```python
from build123d import *

# Parameters (mm, degrees)
F0_W      = 100
F0_H      = 200
F1_DEPTH  = 20
F3_DEPTH  = 10
F5_DEPTH  = 10
F6_R      = 45
F6_R_2    = 30
F7_DEPTH  = 10
F8_R      = 30
F9_DEPTH  = 32
F11_D     = 10
F11_DEPTH = 15
F11_TIP   = 3.0043030951


with BuildPart() as f1:
    # F0 (on Front) → F1 (new body)
    with BuildSketch(Plane.XZ):
        Rectangle(F0_W, F0_H)
    extrude(amount=F1_DEPTH)

    # F2 (on face) → F3 (cut)
    with BuildSketch(Plane(origin=(0, 0, 0), x_dir=(-1, 0, 0), z_dir=(0, 1, 0))):
        with BuildLine():
            ThreePointArc((-28, -60), (-36.4852813742, -63.5147186258), (-40, -72))
            Line((-40, -72), (-40, -78))
            ThreePointArc((-40, -78), (-36.4852813742, -86.4852813742), (-28, -90))
            Line((-28, -90), (28, -90))
            ThreePointArc((28, -90), (36.4852813742, -86.4852813742), (40, -78))
            Line((40, -78), (40, -72))
            ThreePointArc((40, -72), (36.4852813742, -63.5147186258), (28, -60))
            Line((28, -60), (-28, -60))
        make_face()
    extrude(amount=-F3_DEPTH, mode=Mode.SUBTRACT)

    # F4 (on face) → F5 (join)
    with BuildSketch(Plane(origin=(0, 0, 0), x_dir=(-1, 0, 0), z_dir=(0, 1, 0))):
        with BuildLine():
            Line((-48, 45.029), (-48, -38))
            ThreePointArc((-48, -38), (-45.0710678119, -45.0710678119), (-38, -48))
            Line((-38, -48), (38, -48))
            ThreePointArc((38, -48), (45.0710678119, -45.0710678119), (48, -38))
            Line((48, -38), (48, 45.029))
            ThreePointArc((48, 45.029), (47.0866406093, 49.6209930314), (44.4856, 53.5139627365))
            Line((44.4856, 53.5139627365), (10.607, 87.3951071902))
            ThreePointArc((10.607, 87.3951071902), (0, 91.7889037696), (-10.607, 87.3951071902))
            Line((-10.607, 87.3951071902), (-44.4856, 53.5139627365))
            ThreePointArc((-44.4856, 53.5139627365), (-47.0866406093, 49.6209930314), (-48, 45.029))
        make_face()
    extrude(amount=F5_DEPTH)

    # F6 (on face) → F7 (join)
    with BuildSketch(Plane(origin=(0, 10, 0), x_dir=(-1, 0, 0), z_dir=(0, 1, 0))):
        Circle(F6_R)
        Circle(F6_R_2, mode=Mode.SUBTRACT)
        Circle(F6_R_2)
    extrude(amount=F7_DEPTH)

    # F8 (on face) → F9 (cut)
    with BuildSketch(Plane(origin=(0, 20, 0), x_dir=(-1, 0, 0), z_dir=(0, 1, 0))):
        Circle(F8_R)
    extrude(amount=-F9_DEPTH, mode=Mode.SUBTRACT)

    # F11
    with Locations(Plane(origin=(0, 20, 0), x_dir=(-1, 0, 0), z_dir=(0, 1, 0))):
        with Locations((-37.5, 0), (0, 37.5), (0, -37.5), (37.5, 0)):
            Hole(F11_D / 2, depth=F11_DEPTH)
            with Locations((0, 0, -(F11_DEPTH + F11_TIP / 2))):  # 118° drill point
                Cone(0, F11_D / 2, F11_TIP, mode=Mode.SUBTRACT)


solid = f1.part
```
Design review of the part built by this model. Coordinates are the model's own, in mm. A direction names the side the tool comes from. Give positions to 0.01 mm unless a question says otherwise; leave off trailing zeros. Order: outer loops, then holes, each group sorted by start corner. A loop starts at its lowest first (then second) coordinate and runs counter-clockwise, first axis right, second up. Notation, with made-up numbers: (-30, 41) -> (-13, 41) arc R20 ccw to (-13, 50) -> close; hole circle Ø2 at (-29.5, 80.25). An arc over 180 degrees is marked (long way). Write item = value, one per line. Start each with the question number.
(1) We need section C-C on x = 8. Write out the cut boundary in (y, z), plus the area to 3 significant figures.
(2) For pin 1 (2 mm diameter, centred on x = -39, y = 4.5, fed in from -Z); pin 2 (8 mm diameter, centred on y = 4.5, z = -14.5, fed in from -X); pin 3 (1.5 mm diameter, centred on x = 35, z = 43, fed in from +Y); pin 4 (16 mm diameter, centred on x = -37.5, z = 0, fed in from +Y), all flat-tipped, find the tip position at first contact; note any pin that passes through.
(3) For faces 4 (the face through (-47.11, 4.93, 49.56)), 5 (the face through (47.06, 4.93, 49.68)), 6 (the face through (-0.651, 12.395, 42.457)), 7 (the face through (48, 5, 4)), list the 3-axis set-ups (+Z, -Z, +X, -X, +Y, -Y) from which the entire face can be reached by the end or side of a thin tool; tool diameter is ignored.
(4) We need section B-B on z = 71. Write out the cut boundary in (x, y).
(5) To check wall thickness, follow line 1 along Z through (x, y) = (0, 17); line 2 along Z through (x, y) = (0, 9); line 3 along Y through (x, z) = (-17.5, 7). State the ranges of each line that lie inside material, in increasing order.
(6) Mouldability with a two-part tool opening along Z and no side actions: class faces 1 (the face through (-44.99, 4.93, -45.15)), 2 (the face through (-36.39, -4.93, -86.58)), 3 (the face through (1, 10, 54)) as +Z half, -Z half, draft (parallel to the pull), parting line (faces both ways), or undercut.
(7) We need section D-D on z = 23. Write out the cut boundary in (x, y), plus the area to 3 significant figures.
(8) We need section A-A on y = 14.5. Write out the cut boundary in (x, z), plus the area to 3 significant figures.
Numbers:
q1.outline = (-20, -100) -> (0, -100) -> (0, -90) -> (-10, -90) -> (-10, -60) -> (0, -60) -> (0, -48) -> (10, -48) -> (10, -44.28) -> (20, -44.28) -> (20, -28.91) -> (-12, -28.91) -> (-12, 28.91) -> (20, 28.91) -> (20, 44.28) -> (10, 44.28) -> (10, 89.48) -> (0, 89.48) -> (0, 100) -> (-20, 100) -> close
q1.area = 4,110 mm^2
q2.pin_1 = -48
q2.pin_2 = -48
q2.pin_3 = 10
q2.pin_4 = 20
q3.face_4 = +Z, -X, +Y
q3.face_5 = +Z, +X, +Y
q3.face_6 = +Y
q3.face_7 = +Z, -Z, +X, +Y
q4.outline = (-50, -20) -> (50, -20) -> (50, 0) -> (27, 0) -> (27, 10) -> (-27, 10) -> (-27, 0) -> (-50, 0) -> close
q5.line_1 = -45 to -42.5, -32.5 to -30, 30 to 32.5, 42.5 to 45
q5.line_2 = -48 to -42.5, -32.5 to -30, 30 to 32.5, 42.5 to 91.79
q5.line_3 = -20 to -12
q6.face_1 = -Z half
q6.face_2 = undercut
q6.face_3 = draft
q7.outline = (-50, -20) -> (50, -20) -> (50, 0) -> (48, 0) -> (48, 10) -> (38.68, 10) -> (38.68, 20) -> (19.26, 20) -> (19.26, -12) -> (-19.26, -12) -> (-19.26, 20) -> (-38.68, 20) -> (-38.68, 10) -> (-48, 10) -> (-48, 0) -> (-50, 0) -> close
q7.area = 2,500 mm^2
q8.outline = circle Ø90 at (0, 0); hole circle Ø10 at (-37.5, 0); hole circle Ø60 at (0, 0); hole circle Ø10 at (0, -37.5); hole circle Ø10 at (0, 37.5); hole circle Ø10 at (37.5, 0)
q8.area = 3,220 mm^2
